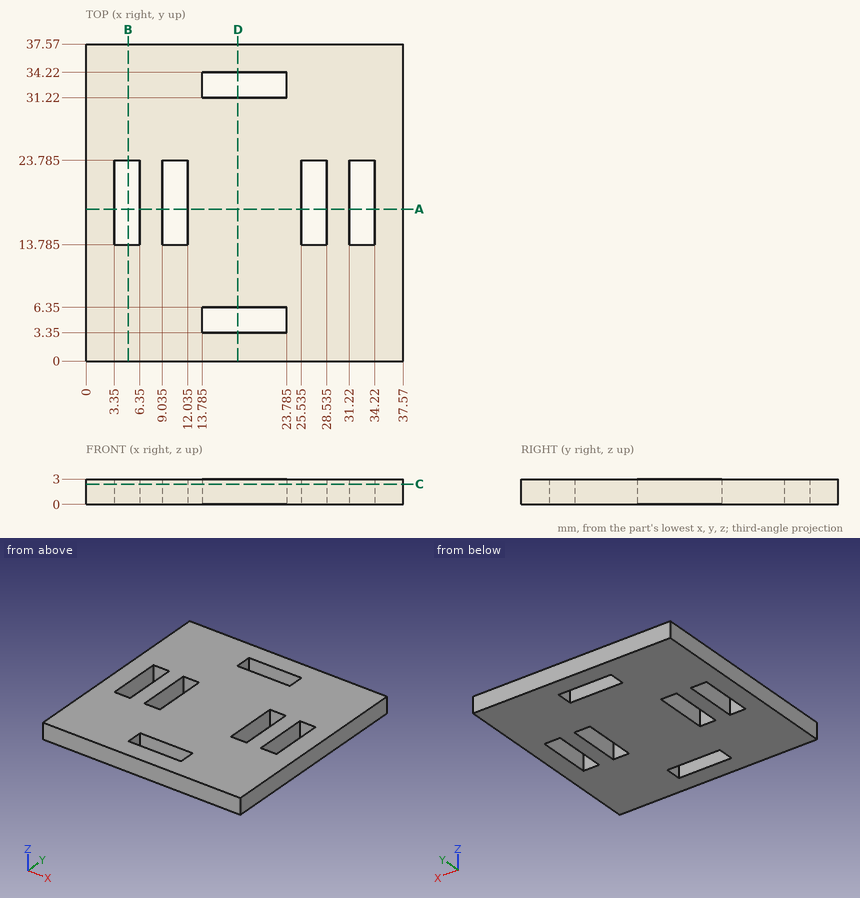
The drawing under review shows one solid part. Ordinate dimensions are in mm from its lowest x, y, z. Coordinates: 2 decimals unless noted, no trailing zeros. Order: outer loops, then holes, each group sorted by start corner. A loop starts at its lowest first (then second) coordinate and runs counter-clockwise, first axis right, second up. Notation, with made-up numbers: (80.5, -38) -> (86.5, -38) arc R19 ccw to (86.5, -10) -> close; hole circle Ø1 at (65.25, 60). An arc over 180 degrees is marked (long way). One line per item, written item: value.
1) We need section A-A, the plane y = 18. Give the boundary of the cut face in (x, z) (3 decimals), then the cut area to 3 significant figures.
Output values:
outline: (0, 0) -> (3.35, 0) -> (3.35, 3) -> (0, 3) -> close; (6.35, 0) -> (9.035, 0) -> (9.035, 3) -> (6.35, 3) -> close; (12.035, 0) -> (25.535, 0) -> (25.535, 3) -> (12.035, 3) -> close; (28.535, 0) -> (31.22, 0) -> (31.22, 3) -> (28.535, 3) -> close; (34.22, 0) -> (37.57, 0) -> (37.57, 3) -> (34.22, 3) -> close
area: 76.7 mm2
2) We need section C-C, the plane z = 2.4. Give the boundary of the cut face in (x, y) (3 decimals).
Output values:
outline: (0, 0) -> (37.57, 0) -> (37.57, 37.57) -> (0, 37.57) -> close; hole (3.35, 13.785) -> (6.35, 13.785) -> (6.35, 23.785) -> (3.35, 23.785) -> close; hole (9.035, 13.785) -> (12.035, 13.785) -> (12.035, 23.785) -> (9.035, 23.785) -> close; hole (13.785, 3.35) -> (23.785, 3.35) -> (23.785, 6.35) -> (13.785, 6.35) -> close; hole (13.785, 31.22) -> (23.785, 31.22) -> (23.785, 34.22) -> (13.785, 34.22) -> close; hole (25.535, 13.785) -> (28.535, 13.785) -> (28.535, 23.785) -> (25.535, 23.785) -> close; hole (31.22, 13.785) -> (34.22, 13.785) -> (34.22, 23.785) -> (31.22, 23.785) -> close
3) We need section B-B, the plane x = 5. Give the boundary of the cut face in (y, z) (3 decimals).
Output values:
outline: (0, 0) -> (13.785, 0) -> (13.785, 3) -> (0, 3) -> close; (23.785, 0) -> (37.57, 0) -> (37.57, 3) -> (23.785, 3) -> close
4) To check wall thickness, follow probe 1 along X at (y, z) = (21.5, 0.6) (3 decimals); probe 2 along Y at (x, z) = (21.5, 0.6); probe 3 along Y at (x, z) = (11, 0.5) (3 decimals). State the ranges of each line that lie inside material, in increasing order. Write a range as [from, to].
Output values:
probe 1: x = [0, 3.35], [6.35, 9.035], [12.035, 25.535], [28.535, 31.22], [34.22, 37.57]
probe 2: y = [0, 3.35], [6.35, 31.22], [34.22, 37.57]
probe 3: y = [0, 13.785], [23.785, 37.57]
5) We need section D-D, the plane x = 18. Give the boundary of the cut face in (y, z).
Output values:
outline: (0, 0) -> (3.35, 0) -> (3.35, 3) -> (0, 3) -> close; (6.35, 0) -> (31.22, 0) -> (31.22, 3) -> (6.35, 3) -> close; (34.22, 0) -> (37.57, 0) -> (37.57, 3) -> (34.22, 3) -> close
